Can you work these out from the model? Positions are in its coordinate system, mm. A direction names the side the tool comes from. Give positions to 0.01 mm unless a question says otherwise; leave off trailing zeros. Write each loop counter-clockwise with the first axis right and the second up, starting at its lowest first coordinate (ties: lowest second). Pieces come first, ordered by that corner, then holes. Notation, with made-up numbers: (-37.75, -14) -> (6.25, -14) arc R15 ccw to (6.25, 4) -> close; hole circle Ø3 at (13, 23). An arc over 180 degrees is marked (long way). One line per item, written item: value.
from build123d import *

# Parameters (mm, degrees)
SKETCH1_R              = 2.5
BOSS_EXTRUDE2_DEPTH    = 5
SPLIT1_SURFACE_1_BACK  = 96.59
SPLIT1_SURFACE_1_DEPTH = 193.18


with BuildPart() as part:
    # Sketch1 → Boss-Extrude2 (new body)
    with BuildSketch(Plane(origin=(0, 0, 0), x_dir=(1, 0, 0), z_dir=(0, 1, 0))):
        with BuildLine():
            Line((47.5, 0), (47.5, -10))
            Line((47.5, -10), (57.5, -10))
            Line((57.5, -10), (57.5, 0))
            ThreePointArc((57.5, 0), (40.658639918, 40.658639918), (0, 57.5))
            Line((0, 57.5), (-10, 57.5))
            Line((-10, 57.5), (-10, 47.5))
            Line((-10, 47.5), (0, 47.5))
            ThreePointArc((0, 47.5), (33.587572106, 33.587572106), (47.5, 0))
        make_face()
        with Locations(Location((52.5, -5, 0), (0, 0, 270))):
            Circle(SKETCH1_R, mode=Mode.SUBTRACT)
        with Locations(Location((-5, 52.5, 0), (0, 0, 90))):
            Circle(SKETCH1_R, mode=Mode.SUBTRACT)
    extrude(amount=BOSS_EXTRUDE2_DEPTH)

    # Split1: cut with a surface, the side behind it stays
    # Split1 surface: a surface, the sketch's curves swept straight by 193.18 mm
    with BuildLine(Plane(origin=(0, 5, 0), x_dir=(1, 0, 0), z_dir=(0, 1, 0)).offset(-SPLIT1_SURFACE_1_BACK), mode=Mode.PRIVATE) as split1_surface_1_path:
        Line((49.32, -10), (49.32, 0))
        ThreePointArc((49.32, 0), (34.874506448, 34.874506448), (0, 49.32))
        Line((0, 49.32), (-10, 49.32))
    split1_surface_1 = Shell.extrude(split1_surface_1_path.wire(), (0 * SPLIT1_SURFACE_1_DEPTH, 1 * SPLIT1_SURFACE_1_DEPTH, 0 * SPLIT1_SURFACE_1_DEPTH))
    split(bisect_by=split1_surface_1, keep=Keep.BOTTOM)


solid = part.part
1) If we section it at C-C (x = 52.5): Write out the boundary of the cut face in (y, z).
Answer list:
outline: (0, -23.45) -> (5, -23.45) -> (5, 2.5) -> (0, 2.5) -> close; (0, 7.5) -> (5, 7.5) -> (5, 10) -> (0, 10) -> close
2) For faces 1 (the face through (-5, 2, -49.32)), 2 (the face through (34, 5, -36)), which set-ups out of +Z, -Z, +X, -X, +Y, -Y let a thin tool reach every point of the face, with its end or its side?
Answer list:
face 1: +Z, -X, +Y, -Y
face 2: +Z, -Z, +X, -X, +Y
3) If we section it at B-B (y = 1.95): Write out the boundary of the cut face in (x, z).
Answer list:
outline: (-10, -57.5) -> (0, -57.5) arc R57.5 ccw to (57.5, 0) -> (57.5, 10) -> (49.32, 10) -> (49.32, 0) arc R49.32 cw to (0, -49.32) -> (-10, -49.32) -> close; hole circle Ø5 at (-5, -52.5); hole circle Ø5 at (52.5, 5)
4) If we section it at D-D (x = 6.5): Write out the boundary of the cut face in (y, z).
Answer list:
outline: (0, -57.13) -> (5, -57.13) -> (5, -48.89) -> (0, -48.89) -> close
5) Will these pins go through, and if not, where does the flat tip stop? pin 1 (3 mm diameter, centred on x = -5, z = -52.5, fed in from +Y); pin 2 (3 mm diameter, centred on y = 1, z = -41, fed in from +X); pin 3 (1.5 mm diameter, centred on y = 3.5, z = -16.5, fed in from -X) (3 decimals); pin 4 (1.5 mm diameter, centred on x = 6, y = 3, fed in from -Z).
Answer list:
pin 1: passes through
pin 2: stops at x = 41.79
pin 3: stops at x = 46.205
pin 4: stops at z = -57.26
6) We'd pull the mould along X, two halves only. Please class faces 3 (the face through (53.251, 2.465, 7.385)), 4 (the face through (57.5, 2, 5)), 5 (the face through (34, 0, -36)): released by +X, released by -X, zero draft, split by the parting line, or undercut.
Answer list:
face 3: undercut
face 4: released by +X
face 5: zero draft
7) If we section it at A-A (z = 5): Write out the boundary of the cut face in (x, y).
Answer list:
outline: (49.32, 0) -> (50, 0) -> (50, 5) -> (49.32, 5) -> close; (55, 0) -> (57.5, 0) -> (57.5, 5) -> (55, 5) -> close
8) I need wall thicknesses on L1, parallel to X at y = 4, z = 5; L2, parallel to Z at x = 51.5, y = 3.55; L3, parallel to X at y = 2.95, z = -52.5. Which ranges of each line are inside material? Lowest first, please.
Answer list:
L1: x = 49.32 to 50, 55 to 57.5
L2: z = -25.57 to 2.71, 7.29 to 10
L3: x = -10 to -7.5, -2.5 to 23.45
